Autodesk Fusion 360 part; units mm, degrees
sketch "Sketch1" plane through (0, 0, 0) normal (0, 0, 1) x (1, 0, 0)
  circle A0 centre (-40.7833, 0) radius 4.25
  circle A1 centre (60.2167, 0) radius 1.65
  circle A2 centre (60.2167, 0) radius 4.25
  circle A3 centre (19.2167, 0) radius 1.65
  circle A4 centre (19.2167, 0) radius 4.25
  circle A5 centre (-40.7833, 0) radius 1.65
  line L0 (-50.7833, -7) -> (70.2167, -7)
  line L1 (70.2167, -7) -> (70.2167, 7)
  line L2 (70.2167, 7) -> (-50.7833, 7)
  line L3 (-50.7833, 7) -> (-50.7833, -7)
  dimension "d3" = 8.5
  dimension "d4" = 3.3
  dimension "d5" = 8.5
  dimension "d6" = 3.3
  dimension "d7" = 8.5
  dimension "d8" = 60
  dimension "d9" = 41
  dimension "d10" = 3.3
  dimension "d11" = 14
  dimension "d12" = 10
  dimension "d13" = 10
  dimension "d14" = 7
extrude "Extrude1" add sketch "Sketch1" along normal blind 2 contours A0 | A2 makes body 1 at (-36.5386, -0.2118, 1.3333) makes body 2 at (64.4614, -0.2118, 1.3333)
extrude "Extrude2" add sketch "Sketch1" along normal blind 4 contours A3 | A4 | L0 L1 L2 L3 bodies 1 2
sketch "Sketch2" plane through (0, 0, 0) normal (0, 1, 0) x (1, 0, 0)
  circle A0 centre (-20.7833, -15.5) radius 1.5
  circle A1 centre (-20.7833, -15.5) radius 4.25
  line L0 (70.2167, 0) -> (-50.7833, 0)
  circle A2 centre (40.2167, -15.5) radius 1.5
  circle A3 centre (40.2167, -15.5) radius 4.25
  line L1 (-28.7833, -23.5) -> (48.2167, -23.5)
  line L2 (48.2167, -23.5) -> (48.2167, -4)
  line L3 (48.2167, -4) -> (-28.7833, -4)
  line L4 (-28.7833, -4) -> (-28.7833, -23.5)
  line L5 (70.2167, -4) -> (-50.7833, -4)
  point P0 (-50.7833, 0)
  point P1 (70.2167, 0)
  dimension "d19" = 3
  dimension "d20" = 8.5
  dimension "d21" = 15.5
  dimension "d22" = 3
  dimension "d23" = 8.5
  dimension "d24" = 15.5
  dimension "d25" = 30
  dimension "d27" = 8
  dimension "d28" = 8
  dimension "d29" = 8
  dimension "d36" = 61
extrude "Extrude3" add sketch "Sketch2" along normal blind 3 from surface at 1 contours L1 L2 L3 L4 L5 bodies 1
extrude "Extrude4" add sketch "Sketch2" along normal blind 2 from surface at 1 contours A1 | A3 bodies 1
chamfer "Chamfer1" distance 8 distance2 9 1 edges at (9.7167, 1, 4) measured on face at (68.3001, 0, 4) on bodies 1
Build history of the part. All positions in model axes, mm. A direction names the side the tool comes from. Give positions to 0.01 mm unless a question says otherwise; leave off trailing zeros. Loops run counter-clockwise (first coordinate to the right, second up) from the corner with the lowest first, then second, coordinate; pieces in that order, holes last.
Item 1: Drill centre lines: line 1 (X direction, y = 3.35, z = 15.5); line 2 (X direction, y = 2.35, z = 15.5); line 3 (Z direction, x = 9.5, y = 6.25). Where is each one in solid material? Low to high.
Answers follow:
line 1: x = -28.78 to -25.03, -16.53 to 35.97, 44.47 to 48.22
line 2: x = -28.78 to -22.28, -19.28 to 38.72, 41.72 to 48.22
line 3: z = 0 to 4
Item 2: Which spindle directions (+Z, -Z, +X, -X, +Y, -Y) get a long thin tool onto all of the face, cutting with end or side? Do faces 1 (the face through (-24.156, 3.493, 12.914)), 2 (the face through (48.217, 1, 12)), 3 (the face through (-28.783, 1, 11)), 4 (the face through (9, 5, 4)), 5 (the face through (9, 1, 18)). Say none if no direction does.
Answers follow:
face 1: +Y
face 2: +Z, +X, +Y, -Y
face 3: +Z, -X, +Y, -Y
face 4: +Z, +Y
face 5: +Z, +X, -X, -Y
Item 3: Slice it at B-B, the plane y = 0. List the corners of the cut face in (x, z), and give its area (3 significant figures).
Answers follow:
outline: (-50.78, 0) - (-42.43, 0) - (-42.43, 2) - (-45.03, 2) - (-45.03, 4) - (-50.78, 4) - close; (-39.13, 0) - (58.57, 0) - (58.57, 2) - (55.97, 2) - (55.97, 4) - (48.22, 4) - (48.22, 11.87) - (-28.78, 11.87) - (-28.78, 4) - (-36.53, 4) - (-36.53, 2) - (-39.13, 2) - close; (61.87, 0) - (70.22, 0) - (70.22, 4) - (64.47, 4) - (64.47, 2) - (61.87, 2) - close
area: 1,040 mm2
Item 4: Slice it at A-A, the plane z = 15.5. List the corners of the cut face in (x, y), and give its area (3 significant figures).
Answers follow:
outline: (-28.78, 1) - (-22.28, 1) - (-22.28, 3) - (-25.03, 3) - (-25.03, 4) - (-28.78, 4) - close; (-19.28, 1) - (38.72, 1) - (38.72, 3) - (35.97, 3) - (35.97, 4) - (-16.53, 4) - (-16.53, 3) - (-19.28, 3) - close; (41.72, 1) - (48.22, 1) - (48.22, 4) - (44.47, 4) - (44.47, 3) - (41.72, 3) - close
area: 202 mm2
Item 5: Flat gauge pins, fed straight in: pin 1 (9.5 mm diameter, centred on x = 38.5, z = 17, fed in from +Y); pin 2 (1 mm diameter, centred on y = 4, z = 9, fed in from +X); pin 3 (4 mm diameter, centred on x = -29.5, z = 6.5, fed in from -Y); pin 4 (2 mm diameter, centred on x = 47.5, y = -5, fed in from -Z). Where does each tip first touch, or does it go through?
Answers follow:
pin 1: stops at y = 4
pin 2: stops at x = 48.22
pin 3: stops at y = -6.44
pin 4: stops at z = 0
Item 6: Pull direction Y, two halves, no side cores. Call faces 6 (the face through (-20.8, 3, 17.3)), 7 (the face through (-50.783, 0, 2)), 8 (the face through (-36.73, -1.28, 2.99)): released by +Y, released by -Y, zero draft, split by the parting line, or undercut.
Answers follow:
face 6: released by +Y
face 7: zero draft
face 8: undercut
Item 7: Slice it at D-D, the plane y = -5.25. List the corners of the cut face in (x, z), and give its area (3 significant figures).
Answers follow:
outline: (-50.78, 0) - (70.22, 0) - (70.22, 4) - (48.22, 4) - (48.22, 5.97) - (-28.78, 5.97) - (-28.78, 4) - (-50.78, 4) - close
area: 635 mm2
